```python
from build123d import *

# Parameters (mm, degrees)
BOSS_EXTRUDE1_DEPTH = 100
SKETCH2_W           = 46.75
SKETCH2_H           = 3
BOSS_EXTRUDE2_DEPTH = 10
SKETCH3_W           = 46.75
SKETCH3_H           = 3
BOSS_EXTRUDE3_DEPTH = 10


with BuildPart() as part:
    # Sketch1 → Boss-Extrude1 (new body)
    with BuildSketch(Plane(origin=(0, 0, 0), x_dir=(1, 0, 0), z_dir=(0, 1, 0))):
        Polygon((0, 6), (0, 0), (-15, 0), (-15, -6), (4.875, -6), (4.875, 15.75), (-5, 15.75), (-5, 6), align=None)
        Polygon((4.875, 15.75), (4.875, -6), (24.75, -6), (31.75, -6), (31.75, 20.5), (29.75, 20.5), (29.75, 14.5), (25.75, 14.5), (25.75, 0), (9.75, 0), (9.75, 6), (14.75, 6), (14.75, 15.75), align=None)
    extrude(amount=BOSS_EXTRUDE1_DEPTH)

    # Sketch2 → Boss-Extrude2 (add)
    with BuildSketch(Plane.XZ):
        with Locations((8.375, 4.5)):
            Rectangle(SKETCH2_W, SKETCH2_H)
    extrude(amount=BOSS_EXTRUDE2_DEPTH)

    # Sketch3 → Boss-Extrude3 (add)
    with BuildSketch(Plane(origin=(0, 100, 0), x_dir=(1, 0, 0), z_dir=(0, 1, 0))):
        with Locations((8.375, -1.5)):
            Rectangle(SKETCH3_W, SKETCH3_H)
    extrude(amount=BOSS_EXTRUDE3_DEPTH)


solid = part.part
```
Part model, mm, in its own coordinate system. A direction names the side the tool comes from. Coordinates: 2 decimals unless noted, no trailing zeros. Write each loop counter-clockwise with the first axis right and the second up, starting at its lowest first coordinate (ties: lowest second). Pieces come first, ordered by that corner, then holes.
Item 1: Mould opens along Z. For faces 1 (the face through (5, 49, -15.75)), 2 (the face through (12, 49, -6)), 3 (the face through (0, 49, -3)), 4 (the face through (14.75, 49, -11)) say: released by +Z, released by -Z, zero draft, split by the parting line, or undercut.
Item 2: Slice it at D-D (z = -18.5). Write the cut outline in (x, y), and give its area (3 significant figures).
Item 3: Slice it at A-A (y = 50). Write the cut outline in (x, z), and give its area (3 significant figures).
Item 4: Probe line 1 (Z direction, x = -3, y = 83); line 2 (X direction, y = 54, z = -7.5); line 3 (X direction, y = 70, z = -1.25). List the from-to ranges inside material, lowest first.
Item 5: Slice it at C-C (x = 27). Write the cut outline in (y, z).
Item 6: Slice it at B-B (z = -8.75). Write the cut outline in (x, y).
Item 7: Pin check, flat tips, straight feed: pin 1 (7 mm diameter, centred on y = 34, z = -7.5, fed in from -X); pin 2 (1 mm diameter, centred on x = 10, z = -11, fed in from +Y); pin 3 (2 mm diameter, centred on x = 15, z = -16.5, fed in from -Y); pin 4 (3 mm diameter, centred on x = -3, z = -17.5, fed in from -Y). Stop position of each tip, or through.
Item 8: Which spindle directions (+Z, -Z, +X, -X, +Y, -Y) get a long thin tool onto all of the face, cutting with end or side? Do faces 5 (the face through (-5, 49, -11)), 6 (the face through (8, 105, 3)), 7 (the face through (9.75, 49, -3)), 8 (the face through (25.75, 49, -7)). Say none if no direction does.
Results found:
1. face 1: released by -Z
1. face 2: undercut
1. face 3: undercut
1. face 4: zero draft
2. outline: (29.75, 0) - (31.75, 0) - (31.75, 100) - (29.75, 100) - close
2. area: 200 mm2
3. outline: (-15, 0) - (0, 0) - (0, -6) - (-5, -6) - (-5, -15.75) - (14.75, -15.75) - (14.75, -6) - (9.75, -6) - (9.75, 0) - (25.75, 0) - (25.75, -14.5) - (29.75, -14.5) - (29.75, -20.5) - (31.75, -20.5) - (31.75, 6) - (-15, 6) - close
3. area: 631 mm2
4. line 1: z = -15.75 to -6, 0 to 6
4. line 2: x = -5 to 14.75, 25.75 to 31.75
4. line 3: x = 0 to 9.75, 25.75 to 31.75
5. outline: (-10, 3) - (0, 3) - (0, -14.5) - (100, -14.5) - (100, 0) - (110, 0) - (110, 3) - (100, 3) - (100, 6) - (-10, 6) - close
6. outline: (-5, 0) - (14.75, 0) - (14.75, 100) - (-5, 100) - close; (25.75, 0) - (31.75, 0) - (31.75, 100) - (25.75, 100) - close
7. pin 1: stops at x = -5
7. pin 2: stops at y = 100
7. pin 3: stops at y = 0
7. pin 4: passes through
8. face 5: -Z, -X, +Y, -Y
8. face 6: +Z, +X, -X, +Y
8. face 7: +Y, -Y
8. face 8: -Z, +Y, -Y
